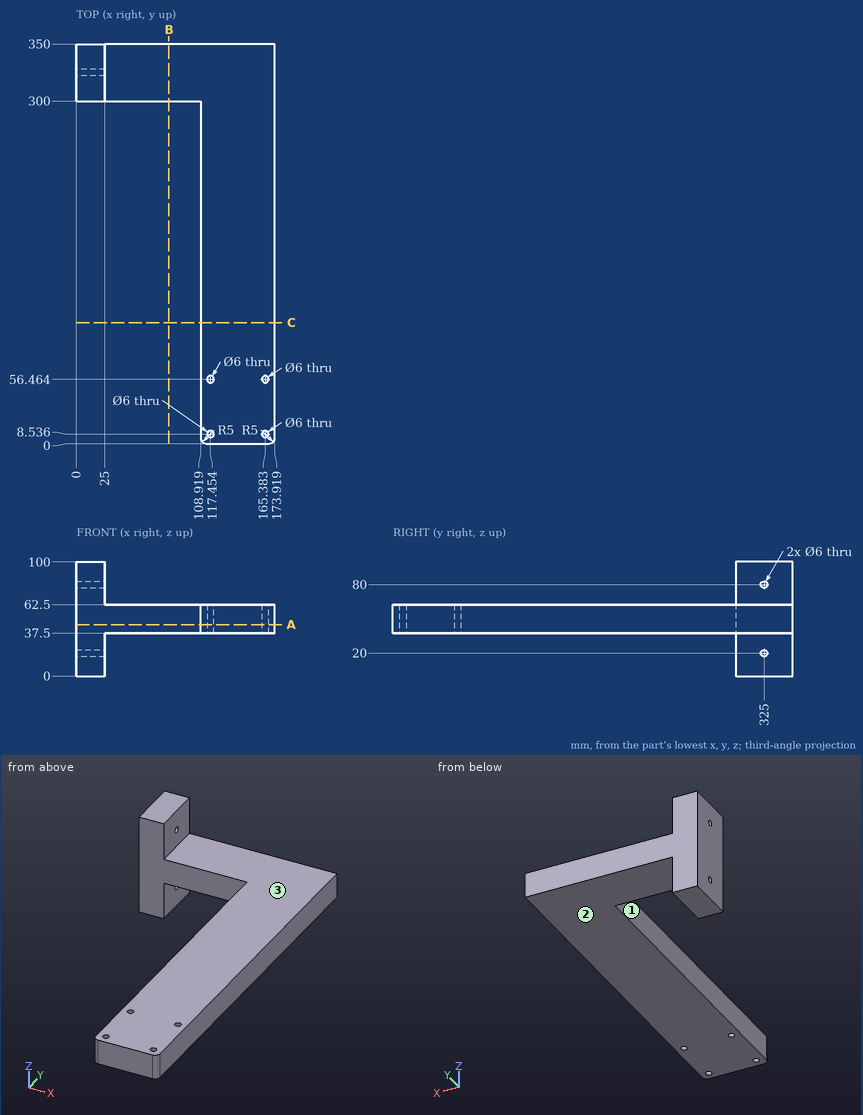
Verification items for this drawing (mm, ordinates from the low corner). A direction names the side the tool comes from. Give positions to 0.01 mm unless a question says otherwise; leave off trailing zeros. Write each loop counter-clockwise with the first axis right and the second up, starting at its lowest first coordinate (ties: lowest second). Pieces come first, ordered by that corner, then holes.
1) Cross-section at C-C (y = 106). Record the boundary of the cut face in (x, z).
Values follow:
outline: (108.92, 37.5) - (173.92, 37.5) - (173.92, 62.5) - (108.92, 62.5) - close
2) Cross-section at B-B (x = 81). Record the boundary of the cut face in (y, z), plus the area to 3 significant figures.
Values follow:
outline: (300, 37.5) - (350, 37.5) - (350, 62.5) - (300, 62.5) - close
area: 1,250 mm2
3) Go/stop test with flat-tipped pins: pin 1 Ø2 at (x, y) = (139, 193) entering from +Z; pin 2 Ø9.5 at (y, z) = (325, 20) entering from +X; pin 3 Ø20 at (y, z) = (83, 54.5) entering from -X; pin 4 Ø5 at (y, z) = (325, 80) entering from -X. Record where each tip stops, or that it passes through.
Values follow:
pin 1: stops at z = 62.5
pin 2: stops at x = 25
pin 3: stops at x = 108.92
pin 4: passes through
4) Cross-section at A-A (z = 45). Record the boundary of the cut face in (x, y) (1 decimal), plus the area to 3 significant figures.
Values follow:
outline: (0, 300) - (108.9, 300) - (108.9, 5) arc R5 ccw to (113.9, 0) - (168.9, 0) arc R5 ccw to (173.9, 5) - (173.9, 350) - (0, 350) - close; hole circle Ø6 at (117.5, 8.5); hole circle Ø6 at (117.5, 56.5); hole circle Ø6 at (165.4, 8.5); hole circle Ø6 at (165.4, 56.5)
area: 28,100 mm2
5) Set-up check for the marked faces 1, 2 and 3: record each of +Z, -Z, +X, -X, +Y, -Y from which the full face is reachable in a straight line by a thin tool's end or side.
Values follow:
face 1: +Z, -Z, -X, -Y
face 2: -Z, +X, +Y, -Y
face 3: +Z, +X, +Y, -Y
6) Thickness scan on line 1 (Z direction, x = 9.5, y = 325); line 2 (Y direction, x = 13, z = 20); line 3 (Z direction, x = 136, y = 86.5). Record the ranges inside material, lowest first.
Values follow:
line 1: z = 0 to 17, 23 to 77, 83 to 100
line 2: y = 300 to 322, 328 to 350
line 3: z = 37.5 to 62.5
